For this review, take the finished solid that the model builds, in its own axes (mm). Give positions to 0.01 mm unless a question says otherwise; leave off trailing zeros. Write each loop counter-clockwise with the first axis right and the second up, starting at its lowest first coordinate (ties: lowest second). Pieces come first, ordered by that corner, then holes. Notation, with made-up numbers: (-29, 89) -> (-11, 89) arc R7 ccw to (-11, 93) -> close; hole circle Ø4 at (18, 15). An arc over 180 degrees is marked (long way). Return JSON: item names as keys, results as strings.
from build123d import *

# Parameters (mm, degrees)
BOX017_W     = 94
BOX017_H     = 158
BOX017_DEPTH = 1
FILLET009_R  = 4
BOX016_W     = 96
BOX016_H     = 162
BOX016_DEPTH = 1
FILLET010_R  = 6
FILLET011_R  = 2


with BuildPart() as fillet009:
    # Box017 → Box017 (new body)
    with BuildSketch(Plane(origin=(26, 6, 116.5), x_dir=(1, 0, 0), z_dir=(0, 0, 1))):
        with Locations((47, 79)):
            Rectangle(BOX017_W, BOX017_H)
    extrude(amount=BOX017_DEPTH)

    # Fillet009
    fillet009_edges = [fillet009.edges().sort_by_distance(p)[0] for p in [
        (120, 6, 117),
        (120, 164, 117),
    ]]
    fillet(fillet009_edges, radius=FILLET009_R)


with BuildPart() as cut352:
    # Box016 → Box016 (new body)
    with BuildSketch(Plane(origin=(26, 4, 116.5), x_dir=(1, 0, 0), z_dir=(0, 0, 1))):
        with Locations((48, 81)):
            Rectangle(BOX016_W, BOX016_H)
    extrude(amount=BOX016_DEPTH)

    # Fillet010
    fillet010_edges = [cut352.edges().sort_by_distance(p)[0] for p in [
        (122, 4, 117),
        (122, 166, 117),
    ]]
    fillet(fillet010_edges, radius=FILLET010_R)

    # Fillet011
    fillet011_edges = [cut352.edges().sort_by_distance(p)[0] for p in [
        (26, 166, 117),
        (26, 4, 117),
    ]]
    fillet(fillet011_edges, radius=FILLET011_R)

    # Cut012: cut Fillet009
    add(fillet009.part, mode=Mode.SUBTRACT)


solid = cut352.part
1. Add section A-A, the plane x = 46. State the section outline as (y, z) points, plus the area to 3 significant figures.
Results found:
{"outline": "(4, 116.5) -> (6, 116.5) -> (6, 117.5) -> (4, 117.5) -> close; (164, 116.5) -> (166, 116.5) -> (166, 117.5) -> (164, 117.5) -> close", "area": "4.00 mm²"}
2. To check wall thickness, follow probe 1 along Y at (x, z) = (77, 116.8); probe 2 along X at (y, z) = (53.5, 116.7). State the ranges of each line that lie inside material, in increasing order.
Results found:
{"probe 1": "y = 4 to 6, 164 to 166", "probe 2": "x = 120 to 122"}
3. Add section B-B, the plane z = 116.9. State the section outline as (x, y) points.
Results found:
{"outline": "(26, 6) arc R2 ccw to (28, 4) -> (116, 4) arc R6 ccw to (122, 10) -> (122, 160) arc R6 ccw to (116, 166) -> (28, 166) arc R2 ccw to (26, 164) -> (116, 164) arc R4 cw to (120, 160) -> (120, 10) arc R4 cw to (116, 6) -> close"}
4. The part is to be moulded in two halves that separate along Y. For faces 1 (the cylindrical face through (120.289, 164.196, 117.007)), 2 (the cylindrical face through (120.196, 5.711, 117.007)), 3 (the cylindrical face through (118.797, 7.141, 117.007)), say which applies: +Y half, -Y half, draft (parallel to the pull), parting line (faces both ways), or undercut.
Results found:
{"face 1": "+Y half", "face 2": "-Y half", "face 3": "undercut"}
5. Add section C-C, the plane y = 38.5. State the section outline as (x, z) points, plus the area to 3 significant figures.
Results found:
{"outline": "(120, 116.5) -> (122, 116.5) -> (122, 117.5) -> (120, 117.5) -> close", "area": "2.00 mm²"}
